Here's how the part is built. I have some questions about the finished solid (model axes, mm). A direction names the side the tool comes from. Round coordinates to 2 decimals unless told otherwise and drop trailing zeros. Order: outer loops, then holes, each group sorted by start corner. A loop starts at its lowest first (then second) coordinate and runs counter-clockwise, first axis right, second up.
```python
from build123d import *

# Parameters (mm, degrees)
EXTRUDE_1_DEPTH          = 22.5
SKETCH_2_W               = 40.1
SKETCH_2_H               = 134.948718637
CUT_EXTRUDE_1_DEPTH      = 6.05
SKETCH_3_W               = 40
SKETCH_3_H               = 54.532079191
CUT_EXTRUDE_2_DEPTH      = 17
CUT_EXTRUDE_3_DEPTH      = 115.04494728
CUT_EXTRUDE_3_DEPTH_BACK = 115.04494728
SKETCH_4_R               = 1.95
SKETCH_5_W               = 28.894932664
SKETCH_5_H               = 60.313820621
SKETCH_5_W_2             = 36.035634414
SKETCH_5_H_2             = 53.811811248
CUT_EXTRUDE_4_DEPTH      = 6.05


with BuildPart() as part:
    # 스케치1 → 보스-돌출1 (new, symmetric)
    with BuildSketch(Plane(origin=(0, 0, 0), x_dir=(0, 0, -1), z_dir=(1, 0, 0))):
        Polygon((0, 0), (34.990619137, 0), (50, 26.923076923), (34.47567302, 76.995358537), (34.47567302, 98.842339146), (33.205617909, 100), (-19.995898679, 56.72140075), (-27.785311637, 14.783172795), align=None)
    extrude(amount=EXTRUDE_1_DEPTH, both=True)

    # 스케치2 → 컷-돌출1 (cut, symmetric)
    with BuildSketch(Plane(origin=(0, 0, 0), x_dir=(0, 0, -1), z_dir=(1, 0, 0))):
        with Locations((8.32658036, 49.272905611)):
            Rectangle(SKETCH_2_W, SKETCH_2_H)
    extrude(amount=CUT_EXTRUDE_1_DEPTH, both=True, mode=Mode.SUBTRACT)

    # 스케치3 → 컷-돌출2 (cut, symmetric)
    with BuildSketch(Plane(origin=(0, 0, 0), x_dir=(0, 0, -1), z_dir=(1, 0, 0))):
        with Locations((8.37658036, 2.733960405)):
            Rectangle(SKETCH_3_W, SKETCH_3_H)
    extrude(amount=CUT_EXTRUDE_2_DEPTH, both=True, mode=Mode.SUBTRACT)

    # 스케치4 → 컷-돌출3 (cut, two sides: drawn at the far end of the back side and taken through both)
    with BuildSketch(Plane(origin=(0, 0, 0), x_dir=(0, 0, -1), z_dir=(1, 0, 0)).offset(-CUT_EXTRUDE_3_DEPTH_BACK)):
        with Locations((-18.546360236, 20)):
            Circle(SKETCH_4_R)
        with Locations((38, 22)):
            Circle(SKETCH_4_R)
    extrude(amount=CUT_EXTRUDE_3_DEPTH + CUT_EXTRUDE_3_DEPTH_BACK, mode=Mode.SUBTRACT)

    # 스케치5 → 컷-돌출4 (cut, symmetric)
    with BuildSketch(Plane(origin=(0, 0, 0), x_dir=(0, 0, -1), z_dir=(1, 0, 0))):
        with Locations((-22.490735836, 15.187792046)):
            Rectangle(SKETCH_5_W, SKETCH_5_H)
        with Locations((41.692548501, 13.265290011)):
            Rectangle(SKETCH_5_W_2, SKETCH_5_H_2)
    extrude(amount=CUT_EXTRUDE_4_DEPTH, both=True, mode=Mode.SUBTRACT)


solid = part.part
```
1. I'm going to push flat-ended pins straight in: P1, Ø3.5, axis at x = 0.5, z = -35, coming from the -Y side; P2, Ø6.5, axis at x = 4, y = 90.5, coming from the -Z side; P3, Ø5, axis at x = -16, z = -36, coming from the +Y side. Where does each tip first touch, or does it pass through?
Evaluation:
P1: stops at y = 40.17
P2: stops at z = -34.48
P3: stops at y = 99.73
2. If we mould it in two halves opening along Y, with no side actions, what happens to faces 4 (the flat face through (12, 15, -28.377)), 5 (the flat face through (18, 0, -21)), 6 (the flat face through (10.315, 36.046, 23.836)), 7 (the cylindrical face through (14.16, 22.59, -39.86))? For each: released by +Y, released by -Y, zero draft, split by the parting line, or undercut.
Evaluation:
face 4: zero draft
face 5: released by -Y
face 6: released by +Y
face 7: undercut
3. If we section it at B-B, the plane y = 55.5: Write out the boundary of the cut face in (x, z).
Evaluation:
outline: (-22.5, -41.14) - (22.5, -41.14) - (22.5, 20.22) - (-22.5, 20.22) - close; hole (-6.05, -28.38) - (6.05, -28.38) - (6.05, 11.72) - (-6.05, 11.72) - close
4. I need wall thicknesses on probe 1 along X at (y, z) = (16, 20); probe 2 along Z at (x, y) = (-12, 20); probe 3 along Z at (x, y) = (-11, 22). Which ranges of each line are inside material? Lowest first, please.
Evaluation:
probe 1: x = -22.5 to -6.05, 6.05 to 22.5
probe 2: z = -46.14 to -28.38, 11.62 to 16.6, 20.5 to 26.82
probe 3: z = -47.26 to -39.95, -36.05 to -28.38, 11.62 to 26.44
5. If we section it at A-A, the plane x = -4: Write out the boundary of the cut face in (y, z).
Evaluation:
outline: (40.17, -45.89) - (77, -34.48) - (98.84, -34.48) - (100, -33.21) - (96.07, -28.38) - (40.17, -28.38) - close; (45.34, 11.72) - (63.45, 11.72) - (56.72, 20) - (45.34, 22.11) - close
6. If we section it at C-C, the plane z = 8: Write out the boundary of the cut face in (x, y), and give its area (3 significant figures).
Evaluation:
outline: (-22.5, 4.26) - (-17, 4.26) - (-17, 30) - (-6.05, 30) - (-6.05, 66.48) - (-22.5, 66.48) - close; (6.05, 30) - (17, 30) - (17, 4.26) - (22.5, 4.26) - (22.5, 66.48) - (6.05, 66.48) - close
area: 1,480 mm2
7. If we section it at D-D, the plane z = -38: Write out the boundary of the cut face in (x, y).
Evaluation:
outline: (-22.5, 5.4) - (-6.05, 5.4) - (-6.05, 20.05) - (-22.5, 20.05) - close; (-22.5, 23.95) - (-6.05, 23.95) - (-6.05, 40.17) - (6.05, 40.17) - (6.05, 23.95) - (22.5, 23.95) - (22.5, 65.63) - (-22.5, 65.63) - close; (6.05, 5.4) - (22.5, 5.4) - (22.5, 20.05) - (6.05, 20.05) - close
8. On a 3-axis mill with a long thin cutter (end or side, diameter ignored), from which of +Z, -Z, +X, -X, +Y, -Y can I reach the whole of each face in a straight line? I mean faces 1 (the flat face through (-18, 0, -21)), 2 (the flat face through (17, 15, -8)), 3 (the flat face through (0, 45.345, 17)). Say none if no direction works.
Evaluation:
face 1: +Z, -Z, +X, -X, -Y
face 2: -Y
face 3: +Z, -Y
